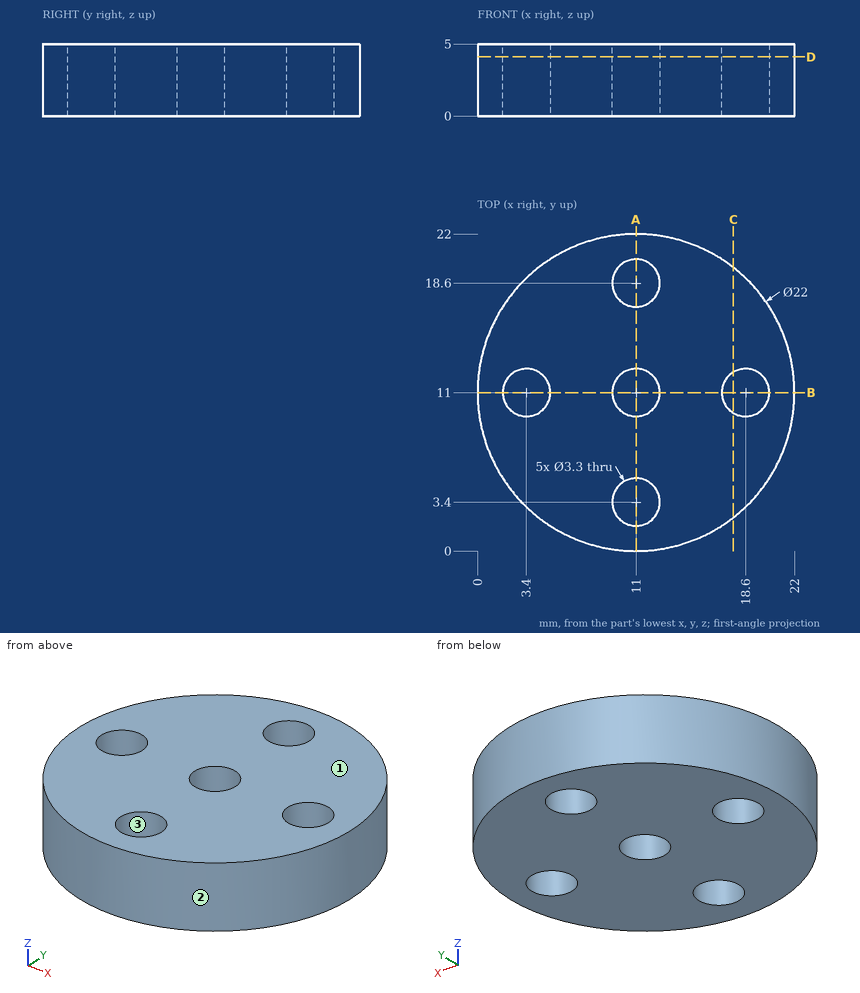
Input: dimensioned drawing with shaded views. Units: mm. Origin: part minimum x, y, z. Coordinates: 2 decimals unless noted, no trailing zeros. Order: outer loops, then holes, each group sorted by start corner. A loop starts at its lowest first (then second) coordinate and runs counter-clockwise, first axis right, second up.
(1) Section query C-C (x = 17.75). Return the cut outline in (y, z), plus the area to 3 significant figures.
(2) Draft query along Y for the marked faces 1, 2 and 3. Return one class per face: pulls with the +Y half, pulls with the -Y half, needs draft (parallel to the pull), parting line crosses it, or undercut.
(3) Section query A-A (x = 11). Return the cut outline in (y, z).
(4) First-contact query: pin 1 (4.5 mm diameter, centred on x = 11, y = 18.6, fed in from +Z); pin 2 (2 mm diameter, centred on y = 14.5, z = 4, fed in from -X); pin 3 (3 mm diameter, centred on x = 15, z = 3, fed in from +Y). Flat tips, straight axial feed; report the tip coordinate or a pass-through.
(5) Material intervals for probe 1 along Y at (x, z) = (11, 2.3); probe 2 along X at (y, z) = (12, 4.05); probe 3 along X at (y, z) = (12.5, 1.6), sorted ascending.
(6) Section query D-D (z = 4.1). Return the cut outline in (x, y).
Solution:
1. outline: (2.31, 0) - (9.59, 0) - (9.59, 5) - (2.31, 5) - close; (12.41, 0) - (19.69, 0) - (19.69, 5) - (12.41, 5) - close
1. area: 72.7 mm2
2. face 1: needs draft
2. face 2: parting line crosses it
2. face 3: undercut
3. outline: (0, 0) - (1.75, 0) - (1.75, 5) - (0, 5) - close; (5.05, 0) - (9.35, 0) - (9.35, 5) - (5.05, 5) - close; (12.65, 0) - (16.95, 0) - (16.95, 5) - (12.65, 5) - close; (20.25, 0) - (22, 0) - (22, 5) - (20.25, 5) - close
4. pin 1: stops at z = 5
4. pin 2: stops at x = 0.29
4. pin 3: stops at y = 21.71
5. probe 1: y = 0 to 1.75, 5.05 to 9.35, 12.65 to 16.95, 20.25 to 22
5. probe 2: x = 0.05 to 2.09, 4.71 to 9.69, 12.31 to 17.29, 19.91 to 21.95
5. probe 3: x = 0.1 to 2.71, 4.09 to 10.31, 11.69 to 17.91, 19.29 to 21.9
6. outline: circle Ø22 at (11, 11); hole circle Ø3.3 at (3.4, 11); hole circle Ø3.3 at (11, 3.4); hole circle Ø3.3 at (11, 11); hole circle Ø3.3 at (11, 18.6); hole circle Ø3.3 at (18.6, 11)
